from build123d import *

# Parameters (mm, degrees)
SKETCH_1_W          = 90
SKETCH_1_H          = 7.85
EXTRUDE_1_DEPTH     = 2
SKETCH_2_W          = 7.85
SKETCH_2_H          = 6
EXTRUDE_2_DEPTH     = 2
SKETCH_3_W          = 7.85
SKETCH_3_H          = 6
EXTRUDE_3_DEPTH     = 2
EXTRUDE_4_DEPTH     = 2
EXTRUDE_5_DEPTH     = 2
EXTRUDE_8_DEPTH     = 1
CUT_EXTRUDE_1_DEPTH = 2.5
EXTRUDE_9_DEPTH     = 3
SKETCH_15_R         = 1.5
CUT_EXTRUDE_2_DEPTH = 3
SKETCH_16_R         = 1.5
CUT_EXTRUDE_3_DEPTH = 3


with BuildPart() as part:
    # 草图1 → 凸台-拉伸1 (new body)
    with BuildSketch(Plane(origin=(0, 0, 0), x_dir=(1, 0, 0), z_dir=(0, 1, 0))):
        with Locations((45, -3.925)):
            Rectangle(SKETCH_1_W, SKETCH_1_H)
    extrude(amount=EXTRUDE_1_DEPTH)

    # 草图2 → 凸台-拉伸2 (add)
    with BuildSketch(Plane(origin=(90, 0, 0), x_dir=(0, 0, -1), z_dir=(1, 0, 0))):
        with Locations((-3.925, 3)):
            Rectangle(SKETCH_2_W, SKETCH_2_H)
    extrude(amount=EXTRUDE_2_DEPTH)

    # 草图3 → 凸台-拉伸3 (add)
    with BuildSketch(Plane.ZY):
        with Locations((3.925, 3)):
            Rectangle(SKETCH_3_W, SKETCH_3_H)
    extrude(amount=EXTRUDE_3_DEPTH)

    # 草图4 → 凸台-拉伸4 (add)
    with BuildSketch(Plane(origin=(0, 0, 0), x_dir=(-1, 0, 0), z_dir=(0, 0, -1))):
        Polygon((2, 0), (2, 6), (0, 6), (-5, 6), (-9, 2), (-9, 0), align=None)
        Polygon((-92, 0), (-92, 6), (-90, 6), (-85, 6), (-81, 2), (-81, 0), align=None)
    extrude(amount=EXTRUDE_4_DEPTH)

    # 草图5 → 凸台-拉伸5 (add)
    with BuildSketch(Plane.XY.offset(7.85)):
        Polygon((92, 0), (92, 6), (90, 6), (86, 2), (86, 0), align=None)
        Polygon((-2, 0), (-2, 6), (0, 6), (4, 2), (4, 0), align=None)
    extrude(amount=EXTRUDE_5_DEPTH)

    # 草图10 → 凸台-拉伸8 (add)
    with BuildSketch(Plane.XZ):
        Polygon((-2, -2), (-2, 9.85), (4, 9.85), (4, 7.85), (86, 7.85), (86, 9.85), (92, 9.85), (92, -2), (81, -2), (81, 0), (9, 0), (9, -2), align=None)
    extrude(amount=EXTRUDE_8_DEPTH)

    # 草图12 → 切除-拉伸1 (cut)
    with BuildSketch(Plane(origin=(0, 2, 0), x_dir=(1, 0, 0), z_dir=(0, 1, 0))):
        Polygon((25.675426481, -3.925), (24.08771324, -1.175), (20.91228676, -1.175), (19.324573519, -3.925), (20.91228676, -6.675), (24.08771324, -6.675), align=None)
        Polygon((70.675426481, -3.925), (69.08771324, -1.175), (65.91228676, -1.175), (64.324573519, -3.925), (65.91228676, -6.675), (69.08771324, -6.675), align=None)
    extrude(amount=-CUT_EXTRUDE_1_DEPTH, mode=Mode.SUBTRACT)

    # 草图13 → 凸台-拉伸9 (add)
    with BuildSketch(Plane(origin=(0, 2, 0), x_dir=(1, 0, 0), z_dir=(0, 1, 0))):
        Polygon((27.984827557, -3.925), (25.242413779, 0.825), (19.757586221, 0.825), (17.015172443, -3.925), (19.757586221, -8.675), (25.242413779, -8.675), align=None)
        Polygon((24.08771324, -6.675), (25.675426481, -3.925), (24.08771324, -1.175), (20.91228676, -1.175), (19.324573519, -3.925), (20.91228676, -6.675), align=None, mode=Mode.SUBTRACT)
        Polygon((72.984827557, -3.925), (70.242413779, 0.825), (64.757586221, 0.825), (62.015172443, -3.925), (64.757586221, -8.675), (70.242413779, -8.675), align=None)
        Polygon((69.08771324, -6.675), (70.675426481, -3.925), (69.08771324, -1.175), (65.91228676, -1.175), (64.324573519, -3.925), (65.91228676, -6.675), align=None, mode=Mode.SUBTRACT)
    extrude(amount=-EXTRUDE_9_DEPTH)

    # 草图15 → 切除-拉伸2 (cut)
    with BuildSketch(Plane(origin=(0, -0.5, 0), x_dir=(1, 0, 0), z_dir=(0, 1, 0))):
        with Locations((22.5, -3.925)):
            Circle(SKETCH_15_R)
    extrude(amount=-CUT_EXTRUDE_2_DEPTH, mode=Mode.SUBTRACT)

    # 草图16 → 切除-拉伸3 (cut)
    with BuildSketch(Plane(origin=(0, -0.5, 0), x_dir=(1, 0, 0), z_dir=(0, 1, 0))):
        with Locations((67.5, -3.925)):
            Circle(SKETCH_16_R)
    extrude(amount=-CUT_EXTRUDE_3_DEPTH, mode=Mode.SUBTRACT)


solid = part.part
Input: part model. Units: mm. Frame: model coordinates. A direction names the side the tool comes from. Give positions to 0.01 mm unless a question says otherwise; leave off trailing zeros. Loops run counter-clockwise (first coordinate to the right, second up) from the corner with the lowest first, then second, coordinate; pieces in that order, holes last. Notation, with made-up numbers: (80.25, -20) -> (105.25, -20) arc R23 cw to (105.25, 18) -> close; hole circle Ø2 at (87.5, 55.5). An arc over 180 degrees is marked (long way). Answer as a JSON object with one key per item and string values. Group by question number.
Item 1: Cut plane B-B, the plane y = 4.5. Return the cut outline in (x, z).
Item 2: Cut plane D-D, the plane y = 1. State how many separate pieces and enclosed holes the cut face has, and give its area (3 significant figures).
Item 3: Reachability of faces 1 (the flat face through (45, 1, 7.85)), 2 (the flat face through (23, 1, 1.175)), 3 (the flat face through (45, 1, 0)) from +Z, -Z, +X, -X, +Y, -Y: full face, straight path, thin tool, end or side. Return the list, or none.
Item 4: Cut plane A-A, the plane x = 67.5. Return the cut outline in (y, z) (3 decimals), and give its area (4 significant figures).
Item 5: Pull-direction query (X, two-part tool) for faces 4 (the flat face through (-2, 3, 4)), 5 (the flat face through (91, 6, 3)), 6 (the flat face through (88, 4, 9)); classes: released by +X, released by -X, zero draft, split by the parting line, or undercut.
Item 6: Line query: probe 1 along X at (y, z) = (1.25, 8.75); probe 2 along X at (y, z) = (5.75, 2); probe 3 along Z at (x, y) = (67.5, -0.8) (3 decimals). Output: solid intervals per line, ascending.
Item 7: Pin query (flat end, axial travel): P1, Ø1.5, axis at x = 74.5, y = 0, coming from the +Z side; P2, Ø0.8, axis at x = 23.5, y = 0.5, coming from the -Z side (3 decimals); P3, Ø2, axis at x = 68, y = 0.5, coming from the +Z side (3 decimals). Return the tip coordinate at first contact, or that it passes through.
Item 8: Cut plane C-C, the plane x = 42. Return the cut outline in (y, z), and give its area (4 significant figures).
Checks:
{
 "1": {"outline": "(-2, -2) -> (6.5, -2) -> (6.5, 0) -> (0, 0) -> (0, 7.85) -> (1.5, 7.85) -> (1.5, 9.85) -> (-2, 9.85) -> close; (83.5, -2) -> (92, -2) -> (92, 9.85) -> (88.5, 9.85) -> (88.5, 7.85) -> (90, 7.85) -> (90, 0) -> (83.5, 0) -> close"},
 "2": {"separate pieces": "1", "enclosed holes": "2", "area": "773 mm²"},
 "3": {"face 1": "+Z, +Y, -Y", "face 2": "+Y", "face 3": "-Z, +Y, -Y"},
 "4": {"outline": "(-1, -0.825) -> (2, -0.825) -> (2, 1.175) -> (-0.5, 1.175) -> (-0.5, 2.425) -> (-1, 2.425) -> close; (-1, 5.425) -> (-0.5, 5.425) -> (-0.5, 6.675) -> (2, 6.675) -> (2, 8.675) -> (-1, 8.675) -> close", "area": "13.25 mm²"},
 "5": {"face 4": "released by -X", "face 5": "zero draft", "face 6": "undercut"},
 "6": {"probe 1": "x = -2 to 4, 86 to 92", "probe 2": "x = -2 to 0, 90 to 92", "probe 3": "z = -0.825 to 2.425, 5.425 to 8.675"},
 "7": {"P1": "stops at z = 7.85", "P2": "stops at z = -0.825", "P3": "stops at z = 8.675"},
 "8": {"outline": "(-1, 0) -> (2, 0) -> (2, 7.85) -> (-1, 7.85) -> close", "area": "23.55 mm²"}
}
